Geometry: see drawing. Coordinates: mm, zero at the bounding-box minimum. Give positions to 0.01 mm unless a question says otherwise; leave off trailing zeros. Order: outer loops, then holes, each group sorted by start corner. A loop starts at its lowest first (then second) coordinate and runs counter-clockwise, first axis right, second up. Notation, with made-up numbers: (17, 30) - (34, 30) arc R20 cw to (34, 47) - close; hole circle Ø8 at (1.5, 26.5). An arc over 180 degrees is marked (long way). One line per item, written item: value. Start each with the question number.
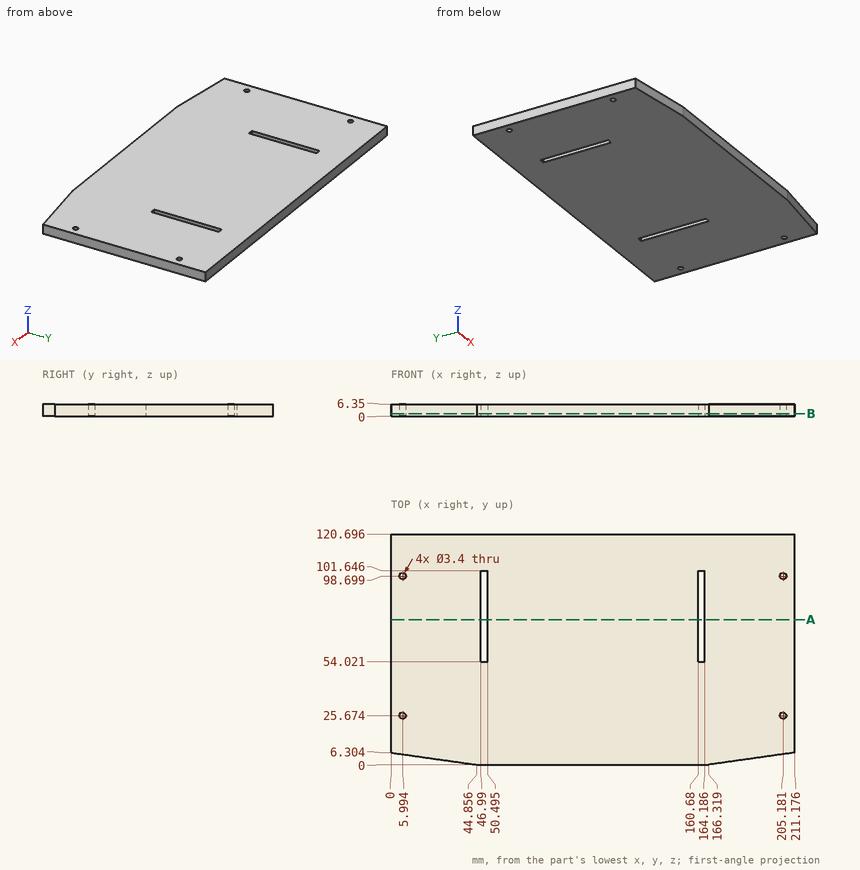
1. Section A-A on y = 76. Count the separate pieces of the cut face and the enclosed holes in it, then the cut area to 3 significant figures.
2. Ray query, L1, parallel to X at y = 88, z = 4.75 (1 decimal); L2, parallel to Y at x = 14, z = 3.25 (1 decimal); L3, parallel to Y at x = 16, z = 5.5 (1 decimal). Return the intervals inside material, ascending.
3. Section B-B on z = 1.25. Return the cut outline in (x, y) (1 decimal).
Data:
1. separate pieces: 3
1. enclosed holes: 0
1. area: 1,300 mm2
2. L1: x = 0 to 47, 50.5 to 160.7, 164.2 to 211.2
2. L2: y = 4.3 to 120.7
2. L3: y = 4.1 to 120.7
3. outline: (0, 6.3) - (44.9, 0) - (166.3, 0) - (211.2, 6.3) - (211.2, 120.7) - (0, 120.7) - close; hole circle Ø3.4 at (6, 25.7); hole circle Ø3.4 at (6, 98.7); hole (47, 54) - (50.5, 54) - (50.5, 101.6) - (47, 101.6) - close; hole (160.7, 54) - (164.2, 54) - (164.2, 101.6) - (160.7, 101.6) - close; hole circle Ø3.4 at (205.2, 25.7); hole circle Ø3.4 at (205.2, 98.7)
